The model under review builds one solid part; all positions refer to its coordinate system, in mm. Face numbers are marked on the shaded views. A direction names the side the tool comes from. Coordinates: 2 decimals unless noted, no trailing zeros. Order: outer loops, then holes, each group sorted by start corner. A loop starts at its lowest first (then second) coordinate and runs counter-clockwise, first axis right, second up. Notation, with made-up numbers: (26.25, -22.5) -> (66.25, -22.5) arc R19 cw to (66.25, -13.5) -> close; hole circle Ø4 at (30.5, 82). An arc over 180 degrees is marked (long way). Put each result on its own line as item: value.
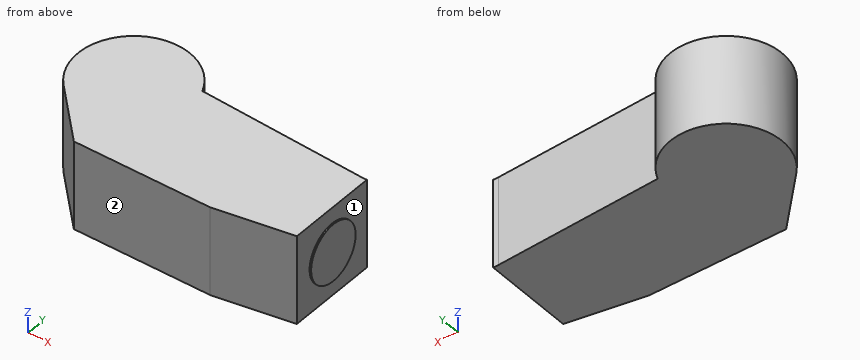
from build123d import *

# Parameters (mm, degrees)
BOSS_EXTRUDE1_DEPTH = 58
SKETCH2_R           = 37.5
BOSS_EXTRUDE2_DEPTH = 2


with BuildPart() as part:
    # Sketch1 → Boss-Extrude1 (new, symmetric)
    with BuildSketch(Plane.XY):
        with BuildLine():
            Line((67, 28.982753492), (284, 17))
            Line((284, 17), (291, 17))
            Line((291, 17), (291, -101))
            Line((291, -101), (191, -118))
            Line((191, -118), (13, -118))
            Line((13, -118), (-52.304922539, -50.92342367))
            ThreePointArc((-52.304922539, -50.92342367), (-40.62309211, 60.652818462), (67, 28.982753492))
        make_face()
    extrude(amount=BOSS_EXTRUDE1_DEPTH, both=True)

    # Sketch2 → Boss-Extrude2 (add)
    with BuildSketch(Plane(origin=(291, 0, 0), x_dir=(0, 0, -1), z_dir=(1, 0, 0))):
        with Locations((0, -42)):
            Circle(SKETCH2_R)
    extrude(amount=BOSS_EXTRUDE2_DEPTH)


solid = part.part
Item 1: Consider section D-D on z = -19. Write out the cut boundary in (x, y), and give its area (3 significant figures).
Answers below:
outline: (-52.3, -50.92) -> (13, -118) -> (191, -118) -> (291, -101) -> (291, -74.33) -> (293, -74.33) -> (293, -9.67) -> (291, -9.67) -> (291, 17) -> (284, 17) -> (67, 28.98) arc R73 ccw (long way) to start
area: 51,700 mm^2
Item 2: For pin 1 Ø3 at (y, z) = (-60, -35.5) entering from -X; pin 2 Ø5 at (y, z) = (15.5, 24.5) entering from -X; pin 3 Ø5.5 at (x, z) = (287, 27) entering from +Y, all flat-tipped, find the tip position at first contact; note any pin that passes through.
Answers below:
pin 1: x = -44.93
pin 2: x = -71.83
pin 3: y = 17
Item 3: For the marked faces 1 and 2, list the 3-axis set-ups (+Z, -Z, +X, -X, +Y, -Y) from which the entire face can be reached by the end or side of a thin tool; tool diameter is ignored.
Answers below:
face 1: +X
face 2: +Z, -Z, +X, -X, -Y
Item 4: Consider section B-B on y = -42. Write out the cut boundary in (x, z), and give its area (3 significant figures).
Answers below:
outline: (-59.71, -58) -> (291, -58) -> (291, -37.5) -> (293, -37.5) -> (293, 37.5) -> (291, 37.5) -> (291, 58) -> (-59.71, 58) -> close
area: 40,800 mm^2
Item 5: Consider section A-A on z = 0. Write out the cut boundary in (x, y).
Answers below:
outline: (-52.3, -50.92) -> (13, -118) -> (191, -118) -> (291, -101) -> (291, -79.5) -> (293, -79.5) -> (293, -4.5) -> (291, -4.5) -> (291, 17) -> (284, 17) -> (67, 28.98) arc R73 ccw (long way) to start
Item 6: For line 1 (Y direction, x = 68, z = -49); line 2 (Y direction, x = 67, z = 38.5); line 3 (X direction, y = 43, z = 35), list the stretches that pass through material, from the lowest coordinate up. Write a range as from..to.
Answers below:
line 1: -118..28.93
line 2: -118..28.98
line 3: -58.99..58.99
Item 7: Consider section C-C on x = 51.5. Write out the cut boundary in (y, z), and give its area (3 significant figures).
Answers below:
outline: (-118, -58) -> (51.74, -58) -> (51.74, 58) -> (-118, 58) -> close
area: 19,700 mm^2
